```python
from build123d import *

# Parameters (mm, degrees)
F1_DEPTH = 13
F2_R     = 1
F3_R     = 1
F4_DEPTH = 25
F5_R     = 1
F6_DEPTH = 25


with BuildPart() as f1:
    # F0 (on Front) → F1 (new body)
    with BuildSketch(Plane.XZ):
        Polygon((-20.602078989, 0), (-18.61380395, 0), (-15.602078989, 0), (-15.602078989, 3), (-5.602078989, 3), (-5.602078989, 0), (-0.602078989, 0), (-0.602078989, 2), (-3.602078989, 2), (-3.602078989, 5), (-17.602078989, 5), (-17.602078989, 2), (-20.602078989, 2), align=None)
    extrude(amount=F1_DEPTH)

    # F2
    f2_edges = [f1.edges().sort_by_distance(p)[0] for p in [
        (-10.602079, 0, 5),
        (-3.602079, -6.5, 5),
        (-17.602079, -6.5, 5),
        (-10.602079, -13, 5),
        (-0.602079, -6.5, 2),
        (-20.602079, -6.5, 2),
    ]]
    fillet(f2_edges, radius=F2_R)

    # F3 (on face) → F4 (cut)
    with BuildSketch(Plane(origin=(0, 0, 0), x_dir=(1, 0, 0), z_dir=(0, 0, -1))):
        with Locations((-18.602078989, 10)):
            Circle(F3_R)
        with Locations((-18.602078989, 3)):
            Circle(F3_R)
    extrude(amount=-F4_DEPTH, mode=Mode.SUBTRACT)

    # F5 (on face) → F6 (cut)
    with BuildSketch(Plane(origin=(0, 0, 0), x_dir=(1, 0, 0), z_dir=(0, 0, -1))):
        with Locations((-2.602078989, 10)):
            Circle(F5_R)
        with Locations((-2.602078989, 3)):
            Circle(F5_R)
    extrude(amount=-F6_DEPTH, mode=Mode.SUBTRACT)


solid = f1.part
```
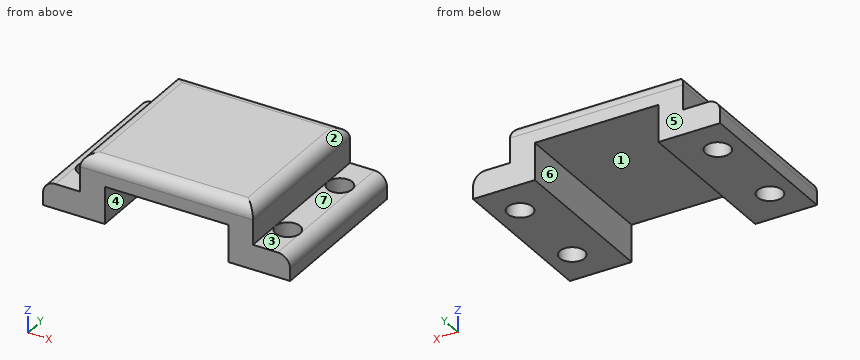
For this review, take the finished solid that the model builds, in its own axes (mm). Face numbers are marked on the shaded views. A direction names the side the tool comes from. Give positions to 0.01 mm unless a question says otherwise; leave off trailing zeros. Order: outer loops, then holes, each group sorted by start corner. A loop starts at its lowest first (then second) coordinate and runs counter-clockwise, first axis right, second up.
1) Take a section at B-B (z = 2.4). Give the boundary of the cut face in (x, y), then the cut area to 3 significant figures.
2) Take a section at A-A (z = 0.7). Give the boundary of the cut face in (x, y).
3) Insertion check: pin 1 (1 mm diameter, centred on y = -6.5, z = 3, fed in from +X); pin 2 (2 mm diameter, centred on x = -19, y = -5, fed in from +Z); pin 3 (1.5 mm diameter, centred on x = -8.5, z = 2.5, fed in from -Y); pin 4 (3 mm diameter, centred on x = -18.6, y = -10, fed in from +Z). Each pin has a flat end and moves straight along its axis. Give the tip position at first contact, or say it passes through.
4) Wall thickness on line 1 (X direction, y = -9.25, z = 2.45); line 2 (X direction, y = -3, z = 1.15); line 3 (X direction, y = -3, z = 1.6): over which ranges is each line inside the solid? List them lowest first.
5) For the marked faces 5, 6 and 7, list the 3-axis set-ups (+Z, -Z, +X, -X, +Y, -Y) from which the entire face can be reached by the end or side of a thin tool; tool diameter is ignored.
6) Take a section at D-D (y = -8). Give the boundary of the cut face in (x, z), then the cut area to 3 significant figures.
7) Take a section at C-C (y = -3.25). State how many separate pieces and enclosed holes the cut face has, then the cut area to 3 significant figures.
8) The part is to be moulded in two halves that separate along X. For the marked faces 1, 2, 3 and 4, say which applies: released by +X, released by -X, zero draft, split by the parting line, or undercut.
Derived:
1. outline: (-17.6, -13) - (-15.6, -13) - (-15.6, 0) - (-17.6, 0) - close; (-5.6, -13) - (-3.6, -13) - (-3.6, 0) - (-5.6, 0) - close
1. area: 52.0 mm2
2. outline: (-20.6, -13) - (-15.6, -13) - (-15.6, 0) - (-20.6, 0) - close; (-5.6, -13) - (-0.6, -13) - (-0.6, 0) - (-5.6, 0) - close; hole circle Ø2 at (-18.6, -10); hole circle Ø2 at (-18.6, -3); hole circle Ø2 at (-2.6, -10); hole circle Ø2 at (-2.6, -3)
3. pin 1: stops at x = -3.6
3. pin 2: stops at z = 2
3. pin 3: stops at y = -13
3. pin 4: stops at z = 4.87
4. line 1: x = -17.6 to -15.6, -5.6 to -3.6
4. line 2: x = -20.59 to -19.6, -17.6 to -15.6, -5.6 to -3.6, -1.6 to -0.61
4. line 3: x = -20.4 to -19.6, -17.6 to -15.6, -5.6 to -3.6, -1.6 to -0.8
5. face 5: +Z, -Z, +X, -X, +Y
5. face 6: -Z, +Y, -Y
5. face 7: +Z, +X, +Y, -Y
6. outline: (-20.6, 0) - (-15.6, 0) - (-15.6, 3) - (-5.6, 3) - (-5.6, 0) - (-0.6, 0) - (-0.6, 1) arc R1 ccw to (-1.6, 2) - (-3.6, 2) - (-3.6, 4) arc R1 ccw to (-4.6, 5) - (-16.6, 5) arc R1 ccw to (-17.6, 4) - (-17.6, 2) - (-19.6, 2) arc R1 ccw to (-20.6, 1) - close
6. area: 51.1 mm2
7. separate pieces: 3
7. enclosed holes: 0
7. area: 43.4 mm2
8. face 1: undercut
8. face 2: released by +X
8. face 3: zero draft
8. face 4: undercut
